Part model, mm, in its own coordinate system. A direction names the side the tool comes from. Give positions to 0.01 mm unless a question says otherwise; leave off trailing zeros. Write each loop counter-clockwise with the first axis right and the second up, starting at its lowest first coordinate (ties: lowest second). Pieces come first, ordered by that corner, then holes.
from build123d import *

# Parameters (mm, degrees)
ESQUISSE1_W             = 40
ESQUISSE1_H             = 40
BOSS_EXTRU_1_DEPTH      = 392
BOSS_EXTRU_2_START      = 50
ESQUISSE2_R             = 10
BOSS_EXTRU_2_DEPTH      = 50
BOSS_EXTRU_2_DRAFT      = 20
ENL_V_MAT_EXTRU_1_DEPTH = 398.882134636


with BuildPart() as part:
    # Esquisse1 → Boss.-Extru.1 (new body)
    with BuildSketch(Plane.XY):
        with Locations((20, 20)):
            Rectangle(ESQUISSE1_W, ESQUISSE1_H)
    extrude(amount=BOSS_EXTRU_1_DEPTH)


with BuildPart() as boss_extru_2_tool:
    # Esquisse2 → Boss.-Extru.2 (with draft: the straight prism first)
    with BuildSketch(Plane.XY.offset(392).offset(BOSS_EXTRU_2_START)):
        with Locations((20, 20)):
            Circle(ESQUISSE2_R)
    extrude(amount=-BOSS_EXTRU_2_DEPTH)
    # Boss.-Extru.2: the draft: its side faces are tilted about the plane it starts from
    boss_extru_2_sides = [boss_extru_2_tool.faces().sort_by_distance(p)[0] for p in [
        (10, 20, 417),
    ]]
    draft(boss_extru_2_sides, Plane.XY.offset(392).offset(BOSS_EXTRU_2_START), BOSS_EXTRU_2_DRAFT)


with BuildPart() as part_1:
    add(part.part)

    # Boss.-Extru.2: add boss_extru_2_tool
    add(boss_extru_2_tool.part)

    # Esquisse3 → Enl_v. mat.-Extru.1 (cut, through all)
    with BuildSketch(Plane(origin=(0, 0, 392), x_dir=(-1, 0, 0), z_dir=(0, 0, -1))):
        with BuildLine():
            ThreePointArc((-0.121467286, 40), (-20, 48.198511713), (-39.878532714, 40))
            Line((-39.878532714, 40), (-0.121467286, 40))
        make_face()
        with BuildLine():
            Line((-40, 0.121467286), (-40, 39.878532714))
            ThreePointArc((-40, 39.878532714), (-48.198511713, 20), (-40, 0.121467286))
        make_face()
        with BuildLine():
            ThreePointArc((0, 0.121467286), (8.198511713, 20), (0, 39.878532714))
            Line((0, 39.878532714), (0, 0.121467286))
        make_face()
        with BuildLine():
            Line((-0.121467286, 0), (-39.878532714, 0))
            ThreePointArc((-39.878532714, 0), (-20, -8.198511713), (-0.121467286, 0))
        make_face()
    extrude(amount=-ENL_V_MAT_EXTRU_1_DEPTH, mode=Mode.SUBTRACT)

    # Esquisse5 → R_volution1 (revolve)
    with BuildSketch(Plane(origin=(20, 0, 0), x_dir=(0, 0, -1), z_dir=(1, 0, 0)), mode=Mode.PRIVATE) as r_volution1_sk:
        Polygon((0, 40), (0, 60), (20, 60), (20, 40), (95, 40), (95, 60), (115, 60), (115, 40), (415, 40), (415, 20), (0, 20), align=None)
    revolve(r_volution1_sk.sketch.rotate(Axis((20, 20, 0), (0, 0, -1)), 180), axis=Axis((20, 20, 0), (0, 0, -1)))


solid = part_1.part
1) Mould opens along Z. For faces 1 (the flat face through (1.7, 29.4, -20)), 2 (the flat face through (0, 20, 204)), 3 (the flat face through (20, 20, -415)) say: +Z half, -Z half, draft (parallel to the pull), parting line (faces both ways), or undercut.
Check result:
face 1: undercut
face 2: draft
face 3: -Z half
2) Flat gauge pins, fed straight in: P1, Ø2, axis at y = 25.5, z = 175, coming from the -X side; P2, Ø1.5, axis at x = 30.5, z = -112.5, coming from the +Y side; P3, Ø4, axis at x = 21, z = 211.5, coming from the +Y side. Where does each tip first touch, or does it go through?
Check result:
P1: stops at x = 0
P2: stops at y = 58.79
P3: stops at y = 40
3) Saw through at C-C (z = -264). Write the cut outline in (x, y), and give its area (3 significant figures).
Check result:
outline: circle Ø40 at (20, 20)
area: 1,260 mm2
4) 3-axis set-ups, long thin cutter, end or side, ignore diameter. For faces 4 (the cylindrical face through (37.743, 10.771, -58.025)), 5 (the cylindrical face through (37.743, 10.771, -267.1)), 6 (the flat face through (20, 40, 204)), 7 (the flat face through (20, 0, 204)), 8 (the flat face through (40, 20, 204)): which of +Z, -Z, +X, -X, +Y, -Y reach the whole face in a straight line?
Check result:
face 4: none
face 5: -Z
face 6: +Z, +X, -X, +Y
face 7: +Z, +X, -X, -Y
face 8: +Z, +X, +Y, -Y
5) Drill centre lines: L1, parallel to Z at x = 33.5, y = -1; L2, parallel to Y at x = 8.5, z = 299.5; L3, parallel to X at y = 26, z = -379.5. Where is each one in solid material? Low to high.
Check result:
L1: z = -115 to -95, -20 to 0
L2: y = 0 to 40
L3: x = 0.92 to 39.08
6) Saw through at A-A (y = 20). Write the cut outline in (x, z).
Check result:
outline: (-20, -115) - (0, -115) - (0, -415) - (40, -415) - (40, -115) - (60, -115) - (60, -95) - (40, -95) - (40, -20) - (60, -20) - (60, 0) - (40, 0) - (40, 414.53) - (30, 442) - (10, 442) - (0, 414.53) - (0, 0) - (-20, 0) - (-20, -20) - (0, -20) - (0, -95) - (-20, -95) - close
